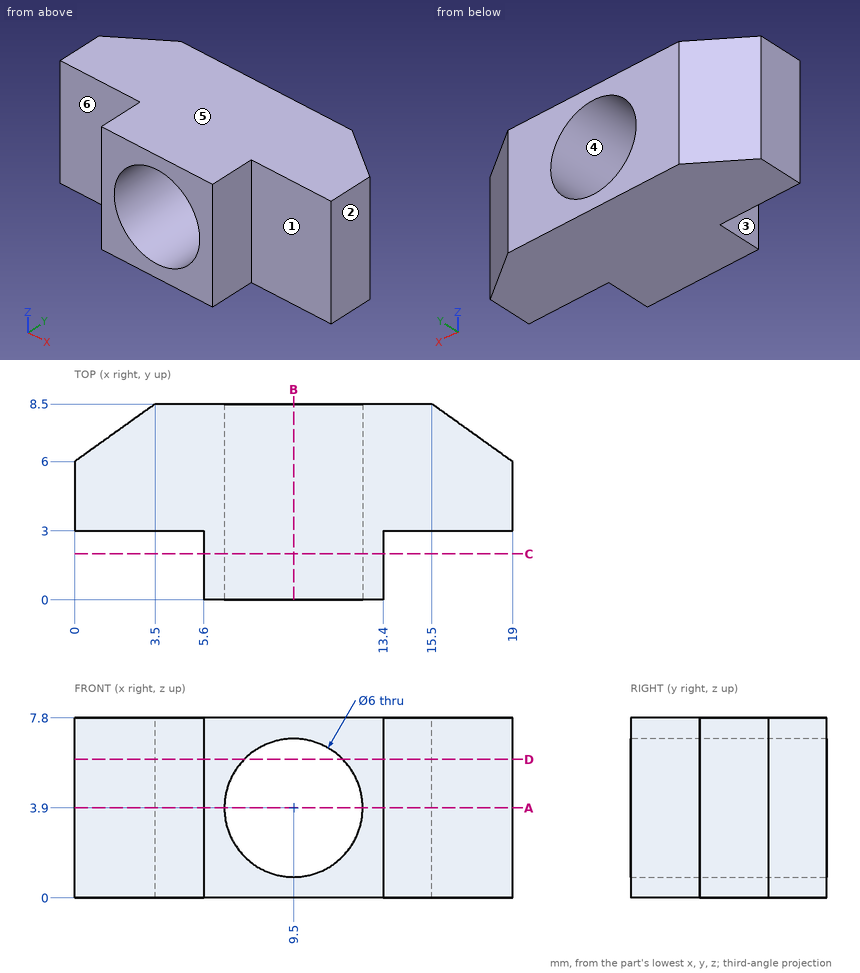
Study the drawing (mm; zero at the part's minimum x, y, z) and answer. A direction names the side the tool comes from. Give positions to 0.01 mm unless a question says otherwise; leave off trailing zeros. Order: outer loops, then holes, each group sorted by start corner. A loop starts at its lowest first (then second) coordinate and runs counter-clockwise, first axis right, second up.
1. Section C-C, the plane y = 2 is taken. Determine the outline of the cut face in (x, z), and give its area (3 significant figures).
Result sheet:
outline: (5.6, 0) - (13.4, 0) - (13.4, 7.8) - (5.6, 7.8) - close; hole circle Ø6 at (9.5, 3.9)
area: 32.6 mm2
2. For the marked faces 1, 2 and 3, determine the directions among +Z, -Z, +X, -X, +Y, -Y from which every point of the face is accessible in a straight line to the end or side of a thin tool.
Result sheet:
face 1: +Z, -Z, +X, -Y
face 2: +Z, -Z, +X, +Y, -Y
face 3: +Z, -Z, -X, -Y
3. Section D-D, the plane z = 6 is taken. Determine the outline of the cut face in (x, y).
Result sheet:
outline: (0, 3) - (5.6, 3) - (5.6, 0) - (7.36, 0) - (7.36, 8.5) - (3.5, 8.5) - (0, 6) - close; (11.64, 0) - (13.4, 0) - (13.4, 3) - (19, 3) - (19, 6) - (15.5, 8.5) - (11.64, 8.5) - close
4. Straight lines are drawn through the part: L1, parallel to X at y = 5.75, z = 3.9; L2, parallel to X at y = 1.5, z = 3.9; L3, parallel to Y at x = 5.5, z = 3.5. For each, find the intervals that lie inside material, in ascending order.
Result sheet:
L1: x = 0 to 6.5, 12.5 to 19
L2: x = 5.6 to 6.5, 12.5 to 13.4
L3: y = 3 to 8.5
5. Each of these flat-tipped pins is pushed along its axis until it touches: P1, Ø1.7, axis at x = 16, z = 2, coming from the -Y side; P2, Ø1.5, axis at y = 2, z = 4, coming from the -X side. Where does it stop, or does it pass through?
Result sheet:
P1: stops at y = 3
P2: stops at x = 5.6
6. Section B-B, the plane x = 9.5 is taken. Determine the outline of the cut face in (y, z), and give its area (3 significant figures).
Result sheet:
outline: (0, 0) - (8.5, 0) - (8.5, 0.9) - (0, 0.9) - close; (0, 6.9) - (8.5, 6.9) - (8.5, 7.8) - (0, 7.8) - close
area: 15.3 mm2
7. Section A-A, the plane z = 3.9 is taken. Determine the outline of the cut face in (x, y).
Result sheet:
outline: (0, 3) - (5.6, 3) - (5.6, 0) - (6.5, 0) - (6.5, 8.5) - (3.5, 8.5) - (0, 6) - close; (12.5, 0) - (13.4, 0) - (13.4, 3) - (19, 3) - (19, 6) - (15.5, 8.5) - (12.5, 8.5) - close
8. The mould has two halves that part along Z. Classify the marked faces 4, 5 and 6: released by +Z, released by -Z, zero draft, split by the parting line, or undercut.
Result sheet:
face 4: undercut
face 5: released by +Z
face 6: zero draft
